Geometry: final body of the model. Coordinates: model frame, mm. Face numbers are marked on the shaded views. A direction names the side the tool comes from. Coordinates: 2 decimals unless noted, no trailing zeros. Loops run counter-clockwise (first coordinate to the right, second up) from the corner with the lowest first, then second, coordinate; pieces in that order, holes last. Notation, with made-up numbers: (21.5, 33.5) - (76.5, 33.5) arc R32 cw to (76.5, 71.5) - close; hole circle Ø10 at (82, -39.5). An arc over 180 degrees is marked (long way). Return JSON: item names as keys, results as strings.
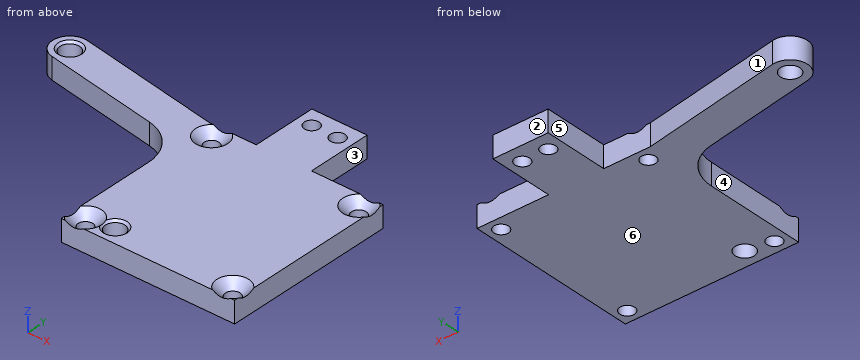
from build123d import *

# Parameters (mm, degrees)
SKETCH1_R           = 1.7
SKETCH1_R_2         = 2.25
BOSS_EXTRUDE1_DEPTH = 5
CHAMFER1_SIZE       = 2
CHAMFER2_SIZE       = 0.5


with BuildPart() as part:
    # Sketch1 → Boss-Extrude1 (new body)
    with BuildSketch(Plane.XY):
        with BuildLine():
            Line((3.5, 20), (3.5, 35))
            Line((3.5, 35), (-9.25, 35))
            Line((-9.25, 35), (-9.25, 20))
            Line((-9.25, 20), (-20, 20))
            Line((-20, 20), (-53.297771938, 25.937877061))
            ThreePointArc((-53.297771938, 25.937877061), (-57.937877061, 22.702228062), (-54.702228062, 18.062122939))
            Line((-54.702228062, 18.062122939), (-28.244429844, 13.343994848))
            ThreePointArc((-28.244429844, 13.343994848), (-22.333328572, 9.919749939), (-20, 3.499302196))
            Line((-20, 3.499302196), (-20, -20))
            Line((-20, -20), (20, -20))
            Line((20, -20), (20, 20))
            Line((20, 20), (3.5, 20))
        make_face()
        with Locations((-17, 17)):
            Circle(SKETCH1_R, mode=Mode.SUBTRACT)
        with Locations((17, 17)):
            Circle(SKETCH1_R, mode=Mode.SUBTRACT)
        with Locations((17, -17)):
            Circle(SKETCH1_R, mode=Mode.SUBTRACT)
        with Locations((-17, -17)):
            Circle(SKETCH1_R, mode=Mode.SUBTRACT)
        with Locations((-5.875, 31)):
            Circle(SKETCH1_R, mode=Mode.SUBTRACT)
        with Locations((0.125, 31)):
            Circle(SKETCH1_R, mode=Mode.SUBTRACT)
        with Locations((-11, -16)):
            Circle(SKETCH1_R_2, mode=Mode.SUBTRACT)
        with Locations((-54, 22)):
            Circle(SKETCH1_R_2, mode=Mode.SUBTRACT)
    extrude(amount=BOSS_EXTRUDE1_DEPTH)

    # Chamfer1
    # the kernel refuses this chamfer: 2 mm, written as the material it takes off along each edge
    with BuildSketch(Plane(origin=(-17, 17, 5), x_dir=(1, 0, 0), z_dir=(0, -1, 0))) as chamfer1_piece_1:
        Polygon((1.7, -CHAMFER1_SIZE), (1.7 + CHAMFER1_SIZE, 0), (1.7, 0), align=None)
    revolve(axis=Axis((-17, 17, 5), (0, 0, 1)), mode=Mode.SUBTRACT)
    with BuildSketch(Plane(origin=(17, 17, 5), x_dir=(1, 0, 0), z_dir=(0, -1, 0))) as chamfer1_piece_2:
        Polygon((1.7, -CHAMFER1_SIZE), (1.7 + CHAMFER1_SIZE, 0), (1.7, 0), align=None)
    revolve(axis=Axis((17, 17, 5), (0, 0, 1)), mode=Mode.SUBTRACT)
    with BuildSketch(Plane(origin=(17, -17, 5), x_dir=(1, 0, 0), z_dir=(0, -1, 0))) as chamfer1_piece_3:
        Polygon((1.7, -CHAMFER1_SIZE), (1.7 + CHAMFER1_SIZE, 0), (1.7, 0), align=None)
    revolve(axis=Axis((17, -17, 5), (0, 0, 1)), mode=Mode.SUBTRACT)
    with BuildSketch(Plane(origin=(-17, -17, 5), x_dir=(1, 0, 0), z_dir=(0, -1, 0))) as chamfer1_piece_4:
        Polygon((1.7, -CHAMFER1_SIZE), (1.7 + CHAMFER1_SIZE, 0), (1.7, 0), align=None)
    revolve(axis=Axis((-17, -17, 5), (0, 0, 1)), mode=Mode.SUBTRACT)

    # Chamfer2
    # the kernel refuses this chamfer: 0.5 mm, written as the material it takes off along each edge
    with BuildSketch(Plane(origin=(-11, -16, 5), x_dir=(1, 0, 0), z_dir=(0, -1, 0))) as chamfer2_piece_1:
        Polygon((2.25 + CHAMFER2_SIZE, 0), (2.25, -CHAMFER2_SIZE), (2.25, 0), align=None)
    revolve(axis=Axis((-11, -16, 5), (0, 0, 1)), mode=Mode.SUBTRACT)
    with BuildSketch(Plane(origin=(-54, 22, 5), x_dir=(1, 0, 0), z_dir=(0, -1, 0))) as chamfer2_piece_2:
        Polygon((2.25 + CHAMFER2_SIZE, 0), (2.25, -CHAMFER2_SIZE), (2.25, 0), align=None)
    revolve(axis=Axis((-54, 22, 5), (0, 0, 1)), mode=Mode.SUBTRACT)


solid = part.part
Item 1: Reachability of the marked faces 1, 2 and 3 from +Z, -Z, +X, -X, +Y, -Y: full face, straight path, thin tool, end or side. Return the list, or none.
Worked out:
{"face 1": "+Z, -Z, +Y", "face 2": "+Z, -Z, +X, -X, +Y", "face 3": "+Z, -Z, +X, +Y"}
Item 2: Section query A-A, the plane x = -17. Return loops of the section in (y, z).
Worked out:
{"outline": "(-20, 0) - (-18.7, 0) - (-18.7, 3) - (-20, 4.3) - close; (-15.3, 0) - (15.3, 0) - (15.3, 3) - (13.3, 5) - (-13.3, 5) - (-15.3, 3) - close; (18.7, 0) - (20, 0) - (20, 4.3) - (18.7, 3) - close"}
Item 3: Section query B-B, the plane y = 22. Return loops of the section in (x, z).
Worked out:
{"outline": "(-58, 0) - (-56.25, 0) - (-56.25, 4.5) - (-56.75, 5) - (-58, 5) - close; (-51.75, 0) - (-31.22, 0) - (-31.22, 5) - (-51.25, 5) - (-51.75, 4.5) - close; (-9.25, 0) - (3.5, 0) - (3.5, 5) - (-9.25, 5) - close"}
Item 4: Ray query, probe 1 along Y at (x, z) = (17, 2.25); probe 2 along X at (y, z) = (30.5, 3.3); probe 3 along Y at (x, z) = (0, 1.2). Return the intervals inside material, ascending. Write a range as from..to.
Worked out:
{"probe 1": "-20..-18.7, -15.3..15.3, 18.7..20", "probe 2": "-9.25..-7.5, -4.25..-1.5, 1.75..3.5", "probe 3": "-20..29.3, 32.7..35"}
Item 5: Section query D-D, the plane y = 9. Return loops of the section in (x, z).
Worked out:
{"outline": "(-21.65, 0) - (20, 0) - (20, 5) - (-21.65, 5) - close"}
Item 6: First-contact query: pin 1 Ø1.5 at (x, z) = (15.5, 1.5) entering from +Y; pin 2 Ø5.5 at (x, y) = (0.125, 31) entering from +Z; pin 3 Ø4 at (x, y) = (-17, -17) entering from +Z. Flat tips, straight axial feed; report the tip coordinate or a pass-through.
Worked out:
{"pin 1": "y = 20", "pin 2": "z = 5", "pin 3": "z = 3.3"}
Item 7: Section query C-C, the plane x = 12. Return loops of the section in (y, z).
Worked out:
{"outline": "(-20, 0) - (20, 0) - (20, 5) - (-20, 5) - close"}
Item 8: Mould query, pull axis X, two halves, no side actions, for the marked faces 4, 5 and 6. Classes: +X half, -X half, draft (parallel to the pull), parting line (faces both ways), or undercut.
Worked out:
{"face 4": "-X half", "face 5": "undercut", "face 6": "draft"}
